CAD build for the part. Positions are in the model's coordinates, mm. A direction names the side the tool comes from. Round coordinates to 2 decimals unless told otherwise and drop trailing zeros. Write each loop counter-clockwise with the first axis right and the second up, starting at its lowest first coordinate (ties: lowest second). Pieces come first, ordered by that corner, then holes. Notation, with made-up numbers: (-16, -2) - (20, -2) arc R23 ccw to (20, 22) - close; hole circle Ø4 at (55, 67.25). An arc over 180 degrees is marked (long way). Put each result on its own line as item: value. Start each with the question number.
Item 1: Cut at A-A (y = -27.75). Give the cut face in (x, z) (3 decimals).
Item 2: 3-axis set-ups, long thin cutter, end or side, ignore diameter. For faces 4 (the cylindrical face through (-12.15, 26.4, -0.25)), 5 (the flat face through (0, -18, -0.5)): which of +Z, -Z, +X, -X, +Y, -Y reach the whole face in a straight line?
Item 3: Cut at D-D (y = -14.5). Give the cut face in (x, z) (3 decimals).
Item 4: Drill centre lines: line 1 (Z direction, x = -7, y = 3); line 2 (Y direction, x = 17, z = 2); line 3 (Y direction, x = 15, z = 5.5). Where is each one in solid material? Low to high. Write a range as from..to.
Item 5: Mould opens along Y. For faces 1 (the cylindrical face through (18.01, 40.95, 3.19)), 2 (the cylindrical face through (-0.92, 26.4, -0.25)), 3 (the flat face through (-11, 22, -0.5)) say: released by +Y, released by -Y, zero draft, split by the parting line, or undercut.
```python
from build123d import *

# Parameters (mm, degrees)
SKETCH_1_W      = 39.45
SKETCH_1_H      = 85.5
EXTRUDE_1_DEPTH = 6.3
FILLET_1_R      = 6
SKETCH_2_R      = 4.25
EXTRUDE_2_DEPTH = 0.5


with BuildPart() as part:
    # 스케치1 → 보스-돌출1 (new body)
    with BuildSketch(Plane.XY):
        Rectangle(SKETCH_1_W, SKETCH_1_H)
    extrude(amount=EXTRUDE_1_DEPTH)

    # 필렛1
    fillet_1_edges = [part.edges().sort_by_distance(p)[0] for p in [
        (19.725, -42.75, 3.15),
        (-19.725, -42.75, 3.15),
        (-19.725, 42.75, 3.15),
        (19.725, 42.75, 3.15),
    ]]
    fillet(fillet_1_edges, radius=FILLET_1_R)

    # 스케치2 → 보스-돌출2 (add)
    with BuildSketch(Plane(origin=(0, 0, 0), x_dir=(-1, 0, 0), z_dir=(0, 0, -1))):
        with Locations(Location((-11.225, 32.25, 0), (0, 0, 180))):
            Circle(SKETCH_2_R)
        with Locations(Location((11.225, 32.25, 0), (0, 0, 180))):
            Circle(SKETCH_2_R)
        with Locations(Location((0, 32.25, 0), (0, 0, 180))):
            Circle(SKETCH_2_R)
        with Locations(Location((-11.225, 22.25, 0), (0, 0, 180))):
            Circle(SKETCH_2_R)
        with Locations(Location((0, 22.25, 0), (0, 0, 180))):
            Circle(SKETCH_2_R)
        with Locations(Location((11.225, 22.25, 0), (0, 0, 180))):
            Circle(SKETCH_2_R)
        with Locations(Location((-11.225, 12.25, 0), (0, 0, 180))):
            Circle(SKETCH_2_R)
        with Locations(Location((0, 12.25, 0), (0, 0, 180))):
            Circle(SKETCH_2_R)
        with Locations(Location((11.225, 12.25, 0), (0, 0, 180))):
            Circle(SKETCH_2_R)
        with Locations(Location((-11.225, 2.25, 0), (0, 0, 180))):
            Circle(SKETCH_2_R)
        with Locations(Location((0, 2.25, 0), (0, 0, 180))):
            Circle(SKETCH_2_R)
        with Locations(Location((11.225, 2.25, 0), (0, 0, 180))):
            Circle(SKETCH_2_R)
        with Locations(Location((-11.225, -7.75, 0), (0, 0, 180))):
            Circle(SKETCH_2_R)
        with Locations(Location((0, -7.75, 0), (0, 0, 180))):
            Circle(SKETCH_2_R)
        with Locations(Location((11.225, -7.75, 0), (0, 0, 180))):
            Circle(SKETCH_2_R)
        with Locations(Location((-11.225, -17.75, 0), (0, 0, 180))):
            Circle(SKETCH_2_R)
        with Locations(Location((0, -17.75, 0), (0, 0, 180))):
            Circle(SKETCH_2_R)
        with Locations(Location((11.225, -17.75, 0), (0, 0, 180))):
            Circle(SKETCH_2_R)
        with Locations(Location((-11.225, -27.75, 0), (0, 0, 180))):
            Circle(SKETCH_2_R)
        with Locations(Location((0, -27.75, 0), (0, 0, 180))):
            Circle(SKETCH_2_R)
        with Locations(Location((11.225, -27.75, 0), (0, 0, 180))):
            Circle(SKETCH_2_R)
    extrude(amount=EXTRUDE_2_DEPTH)


solid = part.part
```
Output values:
1. outline: (-19.725, 0) - (-15.475, 0) - (-15.475, -0.5) - (-6.975, -0.5) - (-6.975, 0) - (-4.25, 0) - (-4.25, -0.5) - (4.25, -0.5) - (4.25, 0) - (6.975, 0) - (6.975, -0.5) - (15.475, -0.5) - (15.475, 0) - (19.725, 0) - (19.725, 6.3) - (-19.725, 6.3) - close
2. face 4: -Z
2. face 5: -Z, +X, -X, +Y, -Y
3. outline: (-19.725, 0) - (-13.964, 0) - (-13.964, -0.5) - (-8.486, -0.5) - (-8.486, 0) - (-2.739, 0) - (-2.739, -0.5) - (2.739, -0.5) - (2.739, 0) - (8.486, 0) - (8.486, -0.5) - (13.964, -0.5) - (13.964, 0) - (19.725, 0) - (19.725, 6.3) - (-19.725, 6.3) - close
4. line 1: 0..6.3
4. line 2: -41.78..41.78
4. line 3: -42.61..42.61
5. face 1: released by +Y
5. face 2: undercut
5. face 3: zero draft
